from build123d import *

# Parameters (mm, degrees)
BOSS_EXTRUDE1_DEPTH = 2.54
SKETCH2_W           = 107.95
SKETCH2_H           = 63.5
CUT_EXTRUDE1_DEPTH  = 226.664855764
CUT_EXTRUDE2_START  = -2.54
CUT_EXTRUDE2_DEPTH  = 2.54


# Read off the part's stored shape, not the designer's step: Cut-Extrude2
with BuildPart() as part:
    # Sketch1 → Boss-Extrude1 (new body)
    with BuildSketch(Plane(origin=(0, 0, 0), x_dir=(1, 0, 0), z_dir=(0, 1, 0))):
        with BuildLine():
            Line((215.9, -14.612459999), (215.9, 36.187540001))
            Line((215.9, 36.187540001), (-215.9, 36.187540001))
            Line((-215.9, 36.187540001), (-215.9, -14.612459999))
            ThreePointArc((-215.9, -14.612459999), (-194.259204241, -52.648965299), (-152.4, -65.412459999))
            Line((-152.4, -65.412459999), (152.4, -65.412459999))
            ThreePointArc((152.4, -65.412459999), (194.259204241, -52.648965299), (215.9, -14.612459999))
        make_face()
    extrude(amount=BOSS_EXTRUDE1_DEPTH)

    # Sketch2 → Cut-Extrude1 (cut, through all)
    with BuildSketch(Plane(origin=(0, 2.54, 0), x_dir=(1, 0, 0), z_dir=(0, 1, 0))):
        with Locations((0, -15.875)):
            Rectangle(SKETCH2_W, SKETCH2_H)
    extrude(amount=-CUT_EXTRUDE1_DEPTH, mode=Mode.SUBTRACT)

    # Cut-Extrude2 outline → Cut-Extrude2 (cut)
    with BuildSketch(Plane(origin=(0, 2.54, 0), x_dir=(1, 0, 0), z_dir=(0, 1, 0)).offset(CUT_EXTRUDE2_START)):
        with BuildLine():
            add(Edge.make_bspline(
                [(-215.899999994, 17.535115527), (-215.566109371, 17.300913161), (-214.20332449, 16.275815014), (-211.81883724, 13.954885046), (-208.930212321, 9.901978384), (-206.463783195, 4.892933776), (-204.667192604, -0.774398824), (-203.719076257, -6.643595697), (-203.665482888, -12.226688771), (-204.419435916, -17.146217321), (-205.817811739, -21.205445303), (-207.685847242, -24.362515926), (-209.864985661, -26.655137817), (-211.469591298, -27.686917669), (-212.297814145, -28.088227647), (-212.355105742, -28.115375011)],
                knots=[0.114839475, 0.114839475, 0.114839475, 0.114839475, 0.125, 0.15625, 0.1875, 0.21875, 0.25, 0.28125, 0.3125, 0.34375, 0.375, 0.40625, 0.4375, 0.46875, 0.471073894, 0.471073894, 0.471073894, 0.471073894], degree=3))
            Line((-215.899999994, 17.535115527), (-215.9, -14.612459999))
            ThreePointArc((-215.9, -14.612459999), (-214.527170136, -21.468828255), (-212.355105742, -28.115375011))
        make_face()
        with BuildLine():
            add(Edge.make_bspline(
                [(212.34685517, -28.136325182), (212.279954773, -28.104999749), (211.441572028, -27.702034349), (209.825715206, -26.66689516), (207.64277821, -24.378244073), (205.76942942, -21.224763186), (204.364219868, -17.16852613), (203.602011314, -12.251147017), (203.646262202, -6.669088999), (204.584578872, -0.799601085), (206.371728131, 4.869386838), (208.829838854, 9.881274858), (211.711764265, 13.937884913), (214.130027538, 16.298772476), (215.528958726, 17.345764848), (215.899999994, 17.602596054)],
                knots=[0.028537672, 0.028537672, 0.028537672, 0.028537672, 0.03125, 0.0625, 0.09375, 0.125, 0.15625, 0.1875, 0.21875, 0.25, 0.28125, 0.3125, 0.34375, 0.375, 0.386307936, 0.386307936, 0.386307936, 0.386307936], degree=3))
            ThreePointArc((212.34685517, -28.136325182), (214.524310397, -21.479717116), (215.9, -14.612459999))
            Line((215.9, -14.612459999), (215.899999994, 17.602596054))
        make_face()
    extrude(amount=CUT_EXTRUDE2_DEPTH, mode=Mode.SUBTRACT)


solid = part.part
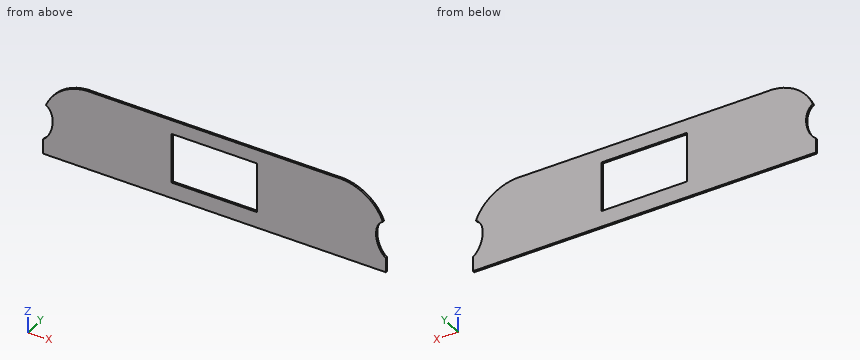
Could you check a few things on this model? Use its own coordinates, in mm. Round coordinates to 2 decimals unless told otherwise and drop trailing zeros. Loops run counter-clockwise (first coordinate to the right, second up) from the corner with the lowest first, then second, coordinate; pieces in that order, holes last. Notation, with made-up numbers: (3.25, 75) -> (41.25, 75) arc R36 cw to (41.25, 112) -> close; hole circle Ø5 at (39.25, 47.25). An arc over 180 degrees is marked (long way). Use CSV: the item, a comma, the result in double quotes.
(1) Suppose I cut it at A-A on z = 34. Write out the boundary of the cut face in (x, y) (3 decimals).
Return value:
outline,"(-209.658, 0) -> (-53.975, 0) -> (-53.975, 2.54) -> (-209.658, 2.54) -> close; (53.975, 0) -> (209.658, 0) -> (209.658, 2.54) -> (53.975, 2.54) -> close"
(2) If I drill on probe 1 along Z at (x, y) = (-31, 1.35) (3 decimals); probe 2 along Z at (x, y) = (-106.5, 0.75); probe 3 along X at (y, z) = (0.5, 45.5) (3 decimals), over which ranges is the centre line in solid material (lowest first)? Write a range as [from, to].
Return value:
probe 1,"z = [-36.188, -15.875], [47.625, 65.412]"
probe 2,"z = [-36.19, 65.41]"
probe 3,"x = [-201.746, -53.975], [53.975, 201.746]"
(3) Will these pins go through, and if not, where does the flat tip stop? pin 1 Ø1.3 at (y, z) = (1, 11) entering from +X; pin 2 Ø1 at (y, z) = (2, 9.5) entering from -X; pin 3 Ø1.5 at (y, z) = (0.5, 26) entering from +X.
Return value:
pin 1,"stops at x = 203.71"
pin 2,"stops at x = -203.73"
pin 3,"stops at x = 210.11"
